```python
from build123d import *

# Parameters (mm, degrees)
SKETCH1_R           = 76.2
SKETCH1_R_2         = 71.12
BOSS_EXTRUDE1_DEPTH = 76.2
SKETCH3_R           = 76.2
BOSS_EXTRUDE2_DEPTH = 6.35
SKETCH4_W           = 63.5
SKETCH4_H           = 63.5
CUT_EXTRUDE1_DEPTH  = 2.54


with BuildPart() as part:
    # Sketch1 → Boss-Extrude1 (new body)
    with BuildSketch(Plane.XY):
        Circle(SKETCH1_R)
        with Locations((0.828825483, 0)):
            Circle(SKETCH1_R_2, mode=Mode.SUBTRACT)
    extrude(amount=BOSS_EXTRUDE1_DEPTH)

    # Sketch3 → Boss-Extrude2 (add)
    with BuildSketch(Plane.XY):
        Circle(SKETCH3_R)
    extrude(amount=BOSS_EXTRUDE2_DEPTH)

    # Sketch4 → Cut-Extrude1 (cut)
    with BuildSketch(Plane.XY.offset(6.35)):
        Rectangle(SKETCH4_W, SKETCH4_H)
    extrude(amount=-CUT_EXTRUDE1_DEPTH, mode=Mode.SUBTRACT)


solid = part.part
```
Check sheet for the modelled part. Datum: model origin and axes. Units: mm. A direction names the side the tool comes from. Round coordinates to 2 decimals unless told otherwise and drop trailing zeros. Order: outer loops, then holes, each group sorted by start corner. A loop starts at its lowest first (then second) coordinate and runs counter-clockwise, first axis right, second up. Notation, with made-up numbers: (50, 33) - (76, 33) arc R18 ccw to (76, 49) - close; hole circle Ø7 at (79, 58). An arc over 180 degrees is marked (long way). Write item = value, one per line.
Q1. Draft check along Y on faces 3 (the face through (-62, -34, 76.2)), 4 (the face through (-60.47, -46.367, 37.567)), 5 (the face through (-14.59, -69.43, 40.79)). Enter one of: pulls with the +Y half, pulls with the -Y half, needs draft (parallel to the pull), parting line crosses it, or undercut.
Computed:
face_3 = needs draft
face_4 = parting line crosses it
face_5 = undercut
Q2. Go/stop test with flat-tipped pins: pin 1 (6 mm diameter, centred on x = -48.5, y = -13.5, fed in from -Z); pin 2 (6 mm diameter, centred on x = -38, z = 21, fed in from -Y); pin 3 (3 mm diameter, centred on x = -14.5, z = 5.5, fed in from -Y); pin 4 (2 mm diameter, centred on y = -12, z = 4.5, fed in from -X). Record where each tip stops, or that it passes through.
Computed:
pin_1 = 0
pin_2 = -67.69
pin_3 = -75.08
pin_4 = -75.4
Q3. Section check C-C (x = -26.5). Record the boundary of the cut face in (y, z).
Computed:
outline = (-71.44, 0) - (71.44, 0) - (71.44, 76.2) - (65.66, 76.2) - (65.66, 6.35) - (31.75, 6.35) - (31.75, 3.81) - (-31.75, 3.81) - (-31.75, 6.35) - (-65.66, 6.35) - (-65.66, 76.2) - (-71.44, 76.2) - close
Q4. Section check D-D (y = 65). Record the boundary of the cut face in (x, z).
Computed:
outline = (-39.77, 0) - (39.77, 0) - (39.77, 76.2) - (29.69, 76.2) - (29.69, 6.35) - (-28.03, 6.35) - (-28.03, 76.2) - (-39.77, 76.2) - close
Q5. Section check A-A (y = 0). Record the boundary of the cut face in (x, z).
Computed:
outline = (-76.2, 0) - (76.2, 0) - (76.2, 76.2) - (71.95, 76.2) - (71.95, 6.35) - (31.75, 6.35) - (31.75, 3.81) - (-31.75, 3.81) - (-31.75, 6.35) - (-70.29, 6.35) - (-70.29, 76.2) - (-76.2, 76.2) - close
Q6. Thickness scan on line 1 along Z through (x, y) = (55.5, 3); line 2 along Z through (x, y) = (12, -1.5); line 3 along X through (y, z) = (54.5, 8.5). Record the ranges inside material, lowest first.
Computed:
line_1 = 0 to 6.35
line_2 = 0 to 3.81
line_3 = -53.26 to -44.86, 46.52 to 53.26
Q7. Section check B-B (z = 22.5). Record the boundary of the cut face in (x, y).
Computed:
outline = circle Ø152.4 at (0, 0); hole circle Ø142.24 at (0.83, 0)
Q8. Tool access check on faces 1 (the face through (-32, 1, 6.35)), 2 (the face through (-1, 1, 0)). Record the directions out of +Z, -Z, +X, -X, +Y, -Y that give a thin tool (end or side, any length) a straight path to the whole face; none if there is none.
Computed:
face_1 = +Z
face_2 = -Z, +X, -X, +Y, -Y
